Design review of the part built by this model. Coordinates are the model's own, in mm. Face numbers are marked on the shaded views. A direction names the side the tool comes from. Coordinates: 2 decimals unless noted, no trailing zeros. Loops run counter-clockwise (first coordinate to the right, second up) from the corner with the lowest first, then second, coordinate; pieces in that order, holes last. Notation, with made-up numbers: M 21.5,32.5 L 60.5,32.5 A22 ccw 60.5,65.5 Z; hole C 27,29.5 d2. An arc over 180 degrees is marked long. Put each result on its own line as item: value. Start each with the question number.
(1) Take a section at D-D, the plane z = 12. Give the boundary of the cut face in (x, y).
(2) Take a section at A-A, the plane z = 20.5. Give the boundary of the cut face in (x, y).
(3) Take a section at B-B, the plane x = 40. Give the boundary of the cut face in (y, z), then the cut area to 3 significant figures.
(4) For probe 1 along X at (y, z) = (1, 20); probe 2 along X at (y, z) = (2, 9); probe 3 along Y at (x, z) = (-43.75, 10.5), list the stretches that pass through material, from the lowest coordinate up. Write a range as [from, to].
(5) For the marked faces 4, 5, 6, 7 and 8, list the 3-axis set-ups (+Z, -Z, +X, -X, +Y, -Y) from which the entire face can be reached by the end or side of a thin tool; tool diameter is ignored.
(6) Clearance check with flat-ended pins moving along their axes: pin 1 (2 mm diameter, centred on y = -13, z = 39, fed in from +X); pin 2 (9.5 mm diameter, centred on x = 0, y = 0, fed in from +Z); pin 3 (19 mm diameter, centred on x = -43.75, y = -23.75, fed in from +Z); pin 4 (10 mm diameter, centred on x = -9, z = 34, fed in from +Y). State where each tip first meets the part, or that it passes through.
(7) Take a section at C-C, the plane x = 0. Give the boundary of the cut face in (y, z), then the cut area to 3 significant figures.
(8) The part is to be moulded in two halves that separate along Z. For the marked faces 1, 2 and 3, say which applies: +Z half, -Z half, draft (parallel to the pull), parting line (faces both ways), or undercut.
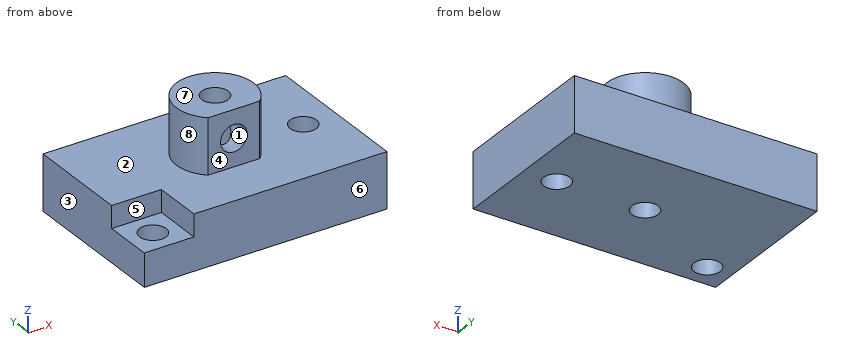
```python
from build123d import *

# Parameters (mm, degrees)
SKETCH_1_W               = 110
SKETCH_1_H               = 70
EXTRUDE_1_DEPTH          = 25
SKETCH_2_R               = 17.5
EXTRUDE_2_DEPTH          = 25
SKETCH_3_R               = 6
CUT_EXTRUDE_1_DEPTH      = 83.158383626
SKETCH_5_W               = 45
SKETCH_5_H               = 45
CUT_EXTRUDE_3_DEPTH      = 10
SKETCH_6_R               = 6
CUT_EXTRUDE_4_DEPTH      = 74.993242935
SKETCH_7_R               = 6
CUT_EXTRUDE_5_DEPTH      = 70.821200219
CUT_EXTRUDE_START        = -25
CUT_EXTRUDE_6_DEPTH      = 25
CUT_EXTRUDE_7_REACH      = 90.482
CUT_EXTRUDE_7_END_RADIUS = 6
SKETCH_9_R               = 6


with BuildPart() as part:
    # Эскиз1 → Бобышка-Вытянуть1 (new body)
    with BuildSketch(Plane.XY):
        Rectangle(SKETCH_1_W, SKETCH_1_H)
    extrude(amount=EXTRUDE_1_DEPTH)

    # Эскиз2 → Бобышка-Вытянуть2 (add)
    with BuildSketch(Plane.XY.offset(25)):
        with Locations(Location((0, 0, 0), (0, 0, 180))):
            Circle(SKETCH_2_R)
    extrude(amount=EXTRUDE_2_DEPTH)

    # Эскиз3 → Вырез-Вытянуть1 (cut, through all)
    with BuildSketch(Plane.XY.offset(50)):
        Circle(SKETCH_3_R)
    extrude(amount=-CUT_EXTRUDE_1_DEPTH, mode=Mode.SUBTRACT)

    # Эскиз5 → Вырез-Вытянуть3 (cut)
    with BuildSketch(Plane.XY.offset(25)):
        with Locations((-55, -35)):
            Rectangle(SKETCH_5_W, SKETCH_5_H)
    extrude(amount=-CUT_EXTRUDE_3_DEPTH, mode=Mode.SUBTRACT)

    # Эскиз6 → Вырез-Вытянуть4 (cut, through all)
    with BuildSketch(Plane.XY.offset(15)):
        with Locations((-43.75, -23.75)):
            Circle(SKETCH_6_R)
    extrude(amount=-CUT_EXTRUDE_4_DEPTH, mode=Mode.SUBTRACT)

    # Эскиз7 → Вырез-Вытянуть5 (cut, through all)
    with BuildSketch(Plane.XY.offset(25)):
        with Locations((40, 0)):
            Circle(SKETCH_7_R)
    extrude(amount=-CUT_EXTRUDE_5_DEPTH, mode=Mode.SUBTRACT)

    # Эскиз8 → Вырез-Вытянуть6 (cut)
    with BuildSketch(Plane.XY.offset(50).offset(CUT_EXTRUDE_START)):
        with BuildLine():
            Line((-11.715374514, -13), (11.715374514, -13))
            ThreePointArc((11.715374514, -13), (0, -17.5), (-11.715374514, -13))
        make_face()
    extrude(amount=CUT_EXTRUDE_6_DEPTH, mode=Mode.SUBTRACT)

    # Вырез-Вытянуть7: up to this cylinder (the profile starts outside it)
    cut_extrude_7_end = Plane(origin=(0, 0, 37.5), z_dir=(0, 0, 1)) * Cylinder(CUT_EXTRUDE_7_END_RADIUS, 193.964, mode=Mode.PRIVATE)
    # Эскиз9 → Вырез-Вытянуть7 (cut, up to the surface)
    with BuildSketch(Plane.XZ.offset(13), mode=Mode.PRIVATE) as cut_extrude_7_sk1:
        with Locations(Location((0, 37.5, 0), (0, 0, 270))):
            Circle(SKETCH_9_R)
    cut_extrude_7_tool1 = extrude(cut_extrude_7_sk1.sketch, amount=-CUT_EXTRUDE_7_REACH, mode=Mode.PRIVATE) - cut_extrude_7_end
    add(cut_extrude_7_tool1.solids().sort_by_distance((0, -13, 37.5))[0], mode=Mode.SUBTRACT)


solid = part.part
```
Computed values:
1. outline: M -55,-35 L 55,-35 L 55,35 L -55,35 Z; hole C -43.75,-23.75 d12; hole C 0,0 d12; hole C 40,0 d12
2. outline: M -55,-12.5 L -32.5,-12.5 L -32.5,-35 L 55,-35 L 55,35 L -55,35 Z; hole C 0,0 d12; hole C 40,0 d12
3. outline: M -35,0 L -6,0 L -6,25 L -35,25 Z; M 6,0 L 35,0 L 35,25 L 6,25 Z
3. area: 1,450 mm^2
4. probe 1: x = [-55, -5.92], [5.92, 34.08], [45.92, 55]
4. probe 2: x = [-55, -5.66], [5.66, 34.34], [45.66, 55]
4. probe 3: y = [-35, -29.75], [-17.75, 35]
5. face 4: +Z, +X, -X, -Y
5. face 5: +Z, -X, -Y
5. face 6: +Z, -Z, +X, -X, -Y
5. face 7: +Z, +X, -X, +Y, -Y
5. face 8: +Z
6. pin 1: stops at x = 12.74
6. pin 2: passes through
6. pin 3: stops at z = 15
6. pin 4: stops at y = 17.04
7. outline: M -35,0 L -6,0 L -6,31.5 L -13,31.5 L -13,25 L -35,25 Z; M -13,43.5 L -6,43.5 L -6,50 L -13,50 Z; M 6,0 L 35,0 L 35,25 L 17.5,25 L 17.5,50 L 6,50 Z
7. area: 1,830 mm^2
8. face 1: undercut
8. face 2: +Z half
8. face 3: draft
